Autodesk Inventor part; units mm, degrees
ref_plane "YZ Plane" through (0, 0, 0) normal (1, 0, 0) x (0, 1, 0)
ref_plane "XZ Plane" through (0, 0, 0) normal (0, 1, 0) x (-1, 0, 0)
ref_plane "XY Plane" through (0, 0, 0) normal (0, 0, 1) x (1, 0, 0)
sketch "Sketch1" plane through (0, 0, 0) normal (0, 1, 0) x (-1, 0, 0)
  line L0 (0, 0) -> (1000, 0)
  line L1 (1000, 0) -> (1000, -1000)
  line L2 (1000, -1000) -> (0, -1000)
  line L3 (0, -1000) -> (0, 0)
  dimension "d0" = 1000
  dimension "d1" = 1000
extrude "Plate1" add sketch "Sketch1" along normal blind 3.048
sketch "Sketch2" plane through (0, 3.048, 0) normal (0, 1, 0) x (1, 0, 0)
  line L0 (-1000, 0) -> (0, 0)
  line L1 (0, 0) -> (-226.9109, 0)
  line L2 (-226.9109, 0) -> (-226.9109, 273.104)
  line L3 (-226.9109, 273.104) -> (0, 273.104)
  line L4 (0, 273.104) -> (0, 0)
  circle A0 centre (-226.9109, 273.104) radius 19.05
  dimension "d3" = 38.1
extrude "Cut1" cut sketch "Sketch2" against normal blind 3.048 contours A0 L3 L2 | L2 L3 A0
sketch "Sketch3" plane through (0, 0, -3.048) normal (0, 0, 1) x (1, 0, 0)
  line L0 (-1000, 0) -> (0, 0)
  line L1 (0, 0) -> (0, 76.2)
  line L2 (0, 76.2) -> (-1000, 76.2)
  line L3 (-1000, 76.2) -> (-1000, 0)
edge flange "Flange1" height 76.2 angle 90 thickness 3.048 bend radius 3.048 thickness toward (0, 0, 1) relief tear relief width 3.048 relief depth 1.524 edges at (-500, 3.048, 0) wall of the first edge with corners at (-1000, 0, -3.048) (0, 0, -3.048) (0, 76.2, -3.048) (-1000, 76.2, -3.048)
bend "Bend1"
corner "Corner1"
sketch "Sketch4" plane through (-1000, 73.152, -3.048) normal (0, 1, 0) x (-1, 0, 0)
  line L0 (-1000, 0) -> (0, 0)
  line L1 (0, 0) -> (0, 76.2)
  line L2 (0, 76.2) -> (-1000, 76.2)
  line L3 (-1000, 76.2) -> (-1000, 0)
edge flange "Flange2" height 76.2 angle 90 thickness 3.048 bend radius 3.048 thickness toward (0, 1, 0) relief tear relief width 3.048 relief depth 1.524 edges at (-500, 76.2, 0) wall of the first edge with corners at (0, 73.152, -3.048) (-1000, 73.152, -3.048) (-1000, 73.152, 73.152) (0, 73.152, 73.152)
bend "Bend2"
corner "Corner2"
sketch "Sketch5" plane through (0, 73.152, 70.104) normal (0, 0, 1) x (1, 0, 0)
  line L0 (-1000, 0) -> (0, 0)
  line L1 (0, 0) -> (0, 76.2)
  line L2 (0, 76.2) -> (-1000, 76.2)
  line L3 (-1000, 76.2) -> (-1000, 0)
edge flange "Flange3" height 76.2 angle 90 thickness 3.048 bend radius 3.048 thickness toward (0, 0, 1) relief tear relief width 3.048 relief depth 1.524 edges at (-500, 76.2, 73.152) wall of the first edge with corners at (-1000, 73.152, 70.104) (0, 73.152, 70.104) (0, 149.352, 70.104) (-1000, 149.352, 70.104)
bend "Bend3"
corner "Corner3"
sketch "Sketch6" plane through (-1000, 146.304, 70.104) normal (0, 1, 0) x (-1, 0, 0)
  line L0 (-1000, 0) -> (0, 0)
  line L1 (0, 0) -> (0, 76.2)
  line L2 (0, 76.2) -> (-1000, 76.2)
  line L3 (-1000, 76.2) -> (-1000, 0)
edge flange "Flange4" height 76.2 angle 90 thickness 3.048 bend radius 3.048 thickness toward (0, 1, 0) relief tear relief width 3.048 relief depth 1.524 edges at (-500, 149.352, 73.152) wall of the first edge with corners at (0, 146.304, 70.104) (-1000, 146.304, 70.104) (-1000, 146.304, 146.304) (0, 146.304, 146.304)
bend "Bend4"
corner "Corner4"
sketch "Sketch7" plane through (0, 146.304, 143.256) normal (0, 0, 1) x (1, 0, 0)
  line L0 (-1000, 0) -> (0, 0)
  line L1 (0, 0) -> (0, 76.2)
  line L2 (0, 76.2) -> (-1000, 76.2)
  line L3 (-1000, 76.2) -> (-1000, 0)
edge flange "Flange5" height 76.2 angle 90 thickness 3.048 bend radius 3.048 thickness toward (0, 0, 1) relief tear relief width 3.048 relief depth 1.524 edges at (-500, 149.352, 146.304) wall of the first edge with corners at (-1000, 146.304, 143.256) (0, 146.304, 143.256) (0, 222.504, 143.256) (-1000, 222.504, 143.256)
bend "Bend5"
corner "Corner5"
sketch "Sketch8" plane through (-1000, 222.504, 146.304) normal (0, 1, 0) x (1, 0, 0)
  point P0 (1000, 146.304)
sketch "Sketch9" plane through (-1000, 219.456, 143.256) normal (0, 1, 0) x (-1, 0, 0)
  line L0 (-1000, 0) -> (0, 0)
  line L1 (0, 0) -> (0, 76.2)
  line L2 (0, 76.2) -> (-1000, 76.2)
  line L3 (-1000, 76.2) -> (-1000, 0)
edge flange "Flange6" height 76.2 angle 90 thickness 3.048 bend radius 3.048 thickness toward (0, 1, 0) relief tear relief width 3.048 relief depth 1.524 edges at (-500, 222.504, 146.304) wall of the first edge with corners at (0, 219.456, 143.256) (-1000, 219.456, 143.256) (-1000, 219.456, 219.456) (0, 219.456, 219.456)
bend "Bend6"
corner "Corner6"
sketch "Sketch10" plane through (0, 219.456, 216.408) normal (0, 0, 1) x (1, 0, 0)
  line L0 (-1000, 0) -> (0, 0)
  line L1 (0, 0) -> (0, 76.2)
  line L2 (0, 76.2) -> (-1000, 76.2)
  line L3 (-1000, 76.2) -> (-1000, 0)
edge flange "Flange7" height 76.2 angle 90 thickness 3.048 bend radius 3.048 thickness toward (0, 0, 1) relief tear relief width 3.048 relief depth 1.524 edges at (-500, 222.504, 219.456) wall of the first edge with corners at (-1000, 219.456, 216.408) (0, 219.456, 216.408) (0, 295.656, 216.408) (-1000, 295.656, 216.408)
bend "Bend7"
corner "Corner7"
equation "\"d4\" = Thickness"
equation "\"d2\" = Thickness"
equation "\"d6\" = BendReliefWidth"
equation "\"d7\" = BendReliefDepth"
equation "\"d8\" = MinimumRemnant"
equation "\"d9\" = TransitionRadius"
equation "\"d12\" = BendRadius"
equation "\"d13\" = CornerReliefSize"
equation "\"d14\" = GapSize"
equation "\"d15\" = JacobiRadiusSize"
equation "\"d16\" = BendReliefWidth"
equation "\"d17\" = BendReliefDepth"
equation "\"d18\" = MinimumRemnant"
equation "\"d19\" = TransitionRadius"
equation "\"d22\" = BendRadius"
equation "\"d23\" = CornerReliefSize"
equation "\"d24\" = GapSize"
equation "\"d25\" = JacobiRadiusSize"
equation "\"d26\" = BendReliefWidth"
equation "\"d27\" = BendReliefDepth"
equation "\"d28\" = MinimumRemnant"
equation "\"d29\" = TransitionRadius"
equation "\"d32\" = BendRadius"
equation "\"d33\" = CornerReliefSize"
equation "\"d34\" = GapSize"
equation "\"d35\" = JacobiRadiusSize"
equation "\"d36\" = BendReliefWidth"
equation "\"d37\" = BendReliefDepth"
equation "\"d38\" = MinimumRemnant"
equation "\"d39\" = TransitionRadius"
equation "\"d42\" = BendRadius"
equation "\"d43\" = CornerReliefSize"
equation "\"d44\" = GapSize"
equation "\"d45\" = JacobiRadiusSize"
equation "\"d46\" = BendReliefWidth"
equation "\"d47\" = BendReliefDepth"
equation "\"d48\" = MinimumRemnant"
equation "\"d49\" = TransitionRadius"
equation "\"d52\" = BendRadius"
equation "\"d53\" = CornerReliefSize"
equation "\"d54\" = GapSize"
equation "\"d55\" = JacobiRadiusSize"
equation "\"d56\" = BendReliefWidth"
equation "\"d57\" = BendReliefDepth"
equation "\"d58\" = MinimumRemnant"
equation "\"d59\" = TransitionRadius"
equation "\"d62\" = BendRadius"
equation "\"d63\" = CornerReliefSize"
equation "\"d64\" = GapSize"
equation "\"d65\" = JacobiRadiusSize"
equation "\"d66\" = BendReliefWidth"
equation "\"d67\" = BendReliefDepth"
equation "\"d68\" = MinimumRemnant"
equation "\"d69\" = TransitionRadius"
equation "\"d72\" = BendRadius"
equation "\"d73\" = CornerReliefSize"
equation "\"d74\" = GapSize"
equation "\"d75\" = JacobiRadiusSize"
equation "\"BendRadius\" = Thickness"
equation "\"BendReliefWidth\" = Thickness"
equation "\"BendReliefDepth\" = 0.5 * Thickness"
equation "\"CornerReliefSize\" = 4 * Thickness"
equation "\"MinimumRemnant\" = 2 * Thickness"
equation "\"TransitionRadius\" = BendRadius"
equation "\"JacobiRadiusSize\" = BendRadius"
equation "\"GapSize\" = Thickness"
properties part number "Floor, Shower" material "Polyethylene, High Density"
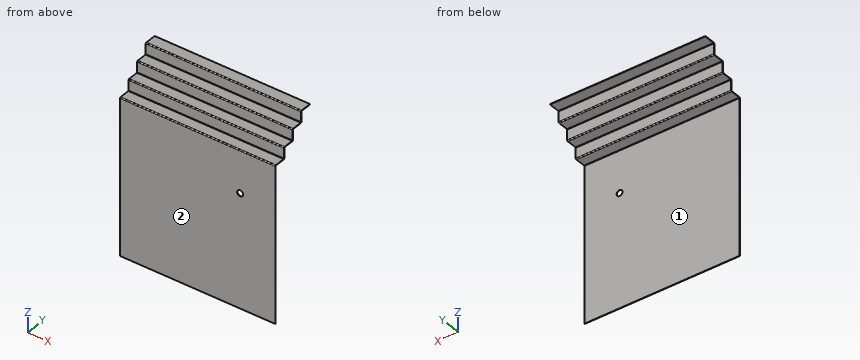
Input: part model. Units: mm. Frame: model coordinates. Face numbers are marked on the shaded views. A direction names the side the tool comes from. Coordinates: 2 decimals unless noted, no trailing zeros. Loops run counter-clockwise (first coordinate to the right, second up) from the corner with the lowest first, then second, coordinate; pieces in that order, holes last. Notation, with made-up numbers: M -24.75,60.25 L 13.25,60.25 A22 ccw 13.25,70.25 Z; hole C -14.5,50.25 d6. An arc over 180 degrees is marked long. Use a Markdown table: item, result. Add a question column.
1) Line query: L1, parallel to Z at x = -101, y = 157.5; L2, parallel to Y at x = -210.5, z = -190; L3, parallel to Z at x = -559.5, y = 22. Output: solid intervals per line, ascending. Write a range as from..to.
2) Section B-B, the plane y = 36. Return the cut outline in (x, z), plus the area to 3 significant figures.
3) Section C-C, the plane z = -134. Return the cut outline in (x, y), plus the area to 3 significant figures.
4) Set-up query: the marked faces 1 and 2. Return all of +Z, -Z, +X, -X, +Y, -Y with unobstructed straight access to the full face (end or side cutting, diameter ignored); none if empty.
5) Pin query (flat end, axial travel): P1, Ø1.5, axis at x = -288.5, y = 130.5, coming from the -Z side; P2, Ø3, axis at x = -660.5, y = 170.5, coming from the +Z side; P3, Ø10, axis at x = -609.5, y = 125, coming from the +Z side. Return the tip coordinate at first contact, or that it passes through.
Answer below:
| question | item | result |
|---|---|---|
| 1 | L1 | 143.26..146.3 |
| 1 | L2 | 0..3.05 |
| 1 | L3 | -3.05..0 |
| 2 | outline | M -1000,-3.05 L 0,-3.05 L 0,0 L -1000,0 Z |
| 2 | area | 3,050 mm2 |
| 3 | outline | M -1000,0 L 0,0 L 0,3.05 L -1000,3.05 Z |
| 3 | area | 3,050 mm2 |
| 4 | face 1 | -Z, +X, -X, +Y |
| 4 | face 2 | +Z, -Z, +X, -X, -Y |
| 5 | P1 | z = 70.1 |
| 5 | P2 | z = 146.3 |
| 5 | P3 | z = 73.15 |
